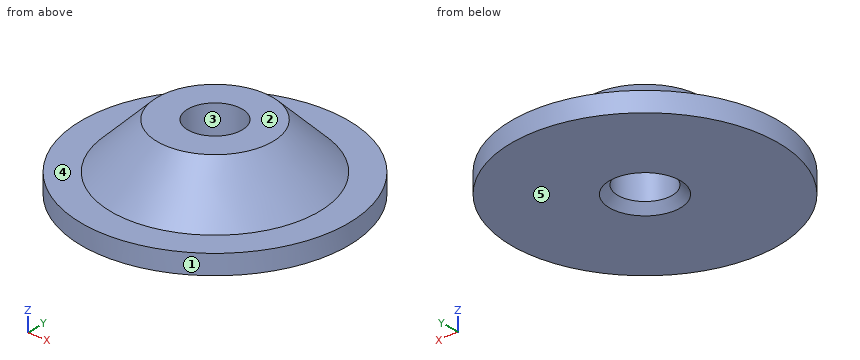
```python
from build123d import *

# Parameters (mm, degrees)
CHAMFER1_SIZE = 0.5


with BuildPart() as part:
    # Sketch3 → Revolve1 (revolve)
    with BuildSketch(Plane(origin=(0, 0, 0), x_dir=(1, 0, 0), z_dir=(0, 1, 0))):
        Polygon((6.3, 0), (8.1, 0), (8.1, 1.2), (1.65, 1.2), (1.65, 0), (1.65, -2.8), (3.5, -2.8), align=None)
    revolve(axis=Axis((0, 0, -35.580076817), (0, 0, 1)))

    # Chamfer1
    chamfer1_edges = [part.edges().sort_by_distance(p)[0] for p in [
        (-1.65, 0, -1.2),
    ]]
    chamfer(chamfer1_edges, length=CHAMFER1_SIZE)


solid = part.part
```
Source: CAD feature listing. Evaluate the final solid. Frame: model axes, mm. Face numbers are marked on the shaded views. A direction names the side the tool comes from. Coordinates: 2 decimals unless noted, no trailing zeros. Loops run counter-clockwise (first coordinate to the right, second up) from the corner with the lowest first, then second, coordinate; pieces in that order, holes last. Notation, with made-up numbers: M 22,22.25 L 72,22.25 A12 ccw 72,36.25 Z; hole C 56.5,24 d10. An arc over 180 degrees is marked long. Put each result on its own line as item: value. Start each with the question number.
1) Cut plane C-C on z = 0.5. Return the cut outline in (x, y), then the cut area to 3 significant figures.
2) Cut plane A-A on y = 0. Return the cut outline in (x, z), then the cut area to 3 significant figures.
3) Pull-direction query (Y, two-part tool) for the marked faces 1, 2 and 3; classes: pulls with the +Y half, pulls with the -Y half, needs draft (parallel to the pull), parting line crosses it, or undercut.
4) Reachability of the marked faces 4 and 5 from +Z, -Z, +X, -X, +Y, -Y: full face, straight path, thin tool, end or side. Return the list, or none.
5) Ray query, L1, parallel to Z at x = -6.5, y = 1.75; L2, parallel to Y at x = 0.5, z = -0.45; L3, parallel to Z at x = 1.5, y = -1. Return the intervals inside material, ascending. Write a range as from..to.
6) Cut plane D-D on y = -7. Return the cut outline in (x, z), then the cut area to 3 significant figures.
7) Contact query for flat-ended pins moving along their axis: pin 1 Ø5.5 at (x, y) = (0, 0) entering from -Z; pin 2 Ø2 at (y, z) = (0, 1.5) entering from +X; pin 3 Ø2 at (x, y) = (6, -4) entering from +Z; pin 4 Ø2 at (y, z) = (-4.5, 1.5) entering from -X. Output: stop coordinate, or through.
The answers:
1. outline: C 0,0 d11.6; hole C 0,0 d3.3
1. area: 97.1 mm²
2. outline: M -8.1,-1.2 L -2.15,-1.2 L -1.65,-0.7 L -1.65,2.8 L -3.5,2.8 L -6.3,0 L -8.1,0 Z; M 1.65,-0.7 L 2.15,-1.2 L 8.1,-1.2 L 8.1,0 L 6.3,0 L 3.5,2.8 L 1.65,2.8 Z
2. area: 33.4 mm²
3. face 1: parting line crosses it
3. face 2: needs draft
3. face 3: undercut
4. face 4: +Z
4. face 5: -Z, +X, -X, +Y, -Y
5. L1: z = -1.2..0
5. L2: y = -8.08..-1.57, 1.57..8.08
5. L3: z = -0.85..2.8
6. outline: M -4.08,-1.2 L 4.08,-1.2 L 4.08,0 L -4.08,0 Z
6. area: 9.78 mm²
7. pin 1: stops at z = -1.2
7. pin 2: stops at x = 5.8
7. pin 3: stops at z = 0.09
7. pin 4: stops at x = -4.02
